Geometry: see drawing. Coordinates: mm, zero at the bounding-box minimum. Coordinates: 2 decimals unless noted, no trailing zeros. Write each loop counter-clockwise with the first axis right and the second up, starting at its lowest first coordinate (ties: lowest second). Pieces come first, ordered by that corner, then holes. Notation, with made-up numbers: M 39,47 L 73,47 A21 cw 73,82 Z; hole C 39.25,51.5 d3. An arc over 180 degrees is marked long. Write item = value, one per line. Start each with the question number.
1. Pin query (flat end, axial travel): pin 1 Ø1.9 at (x, z) = (8, 3.5) entering from +Y; pin 2 Ø1.9 at (y, z) = (1.5, 4) entering from -X; pin 3 Ø1.9 at (y, z) = (62, 3) entering from +X. Return the tip coordinate at first contact, or that it passes through.
2. Section query B-B (y = 31). Output: boundary loops of the cut face in (x, z), then the cut area to 3 significant figures.
3. Line query: line 1 along Y through (x, z) = (155.5, 3.25); line 2 along Y through (x, z) = (16, 4); line 3 along X through (y, z) = (18, 4.75). Output: solid intervals per line, ascending.
4. Section query C-C (y = 62). Output: boundary loops of the cut face in (x, z), then the cut area to 3 significant figures.
5. Section query A-A (z = 1). Output: boundary loops of the cut face in (x, y), then the cut area to 3 significant figures.
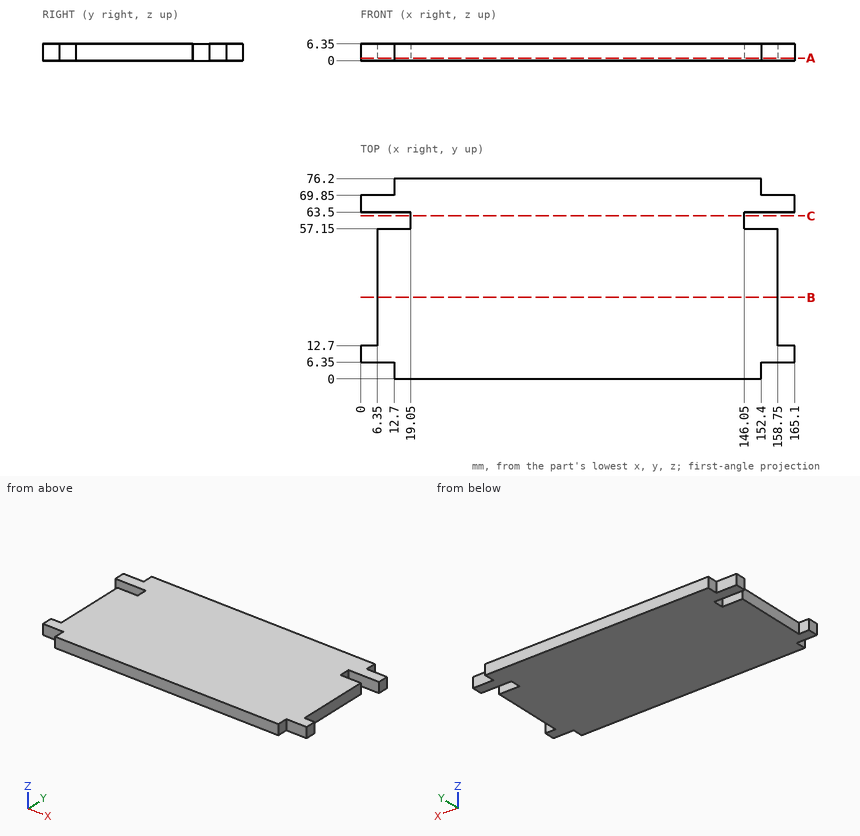
Results are:
q1.pin_1 = 69.85
q1.pin_2 = 12.7
q1.pin_3 = 146.05
q2.outline = M 6.35,0 L 158.75,0 L 158.75,6.35 L 6.35,6.35 Z
q2.area = 968 mm^2
q3.line_1 = 6.35 to 57.15, 63.5 to 69.85
q3.line_2 = 0 to 57.15, 63.5 to 76.2
q3.line_3 = 6.35 to 158.75
q4.outline = M 19.05,0 L 146.05,0 L 146.05,6.35 L 19.05,6.35 Z
q4.area = 806 mm^2
q5.outline = M 0,6.35 L 12.7,6.35 L 12.7,0 L 152.4,0 L 152.4,6.35 L 165.1,6.35 L 165.1,12.7 L 158.75,12.7 L 158.75,57.15 L 146.05,57.15 L 146.05,63.5 L 165.1,63.5 L 165.1,69.85 L 152.4,69.85 L 152.4,76.2 L 12.7,76.2 L 12.7,69.85 L 0,69.85 L 0,63.5 L 19.05,63.5 L 19.05,57.15 L 6.35,57.15 L 6.35,12.7 L 0,12.7 Z
q5.area = 11,500 mm^2
